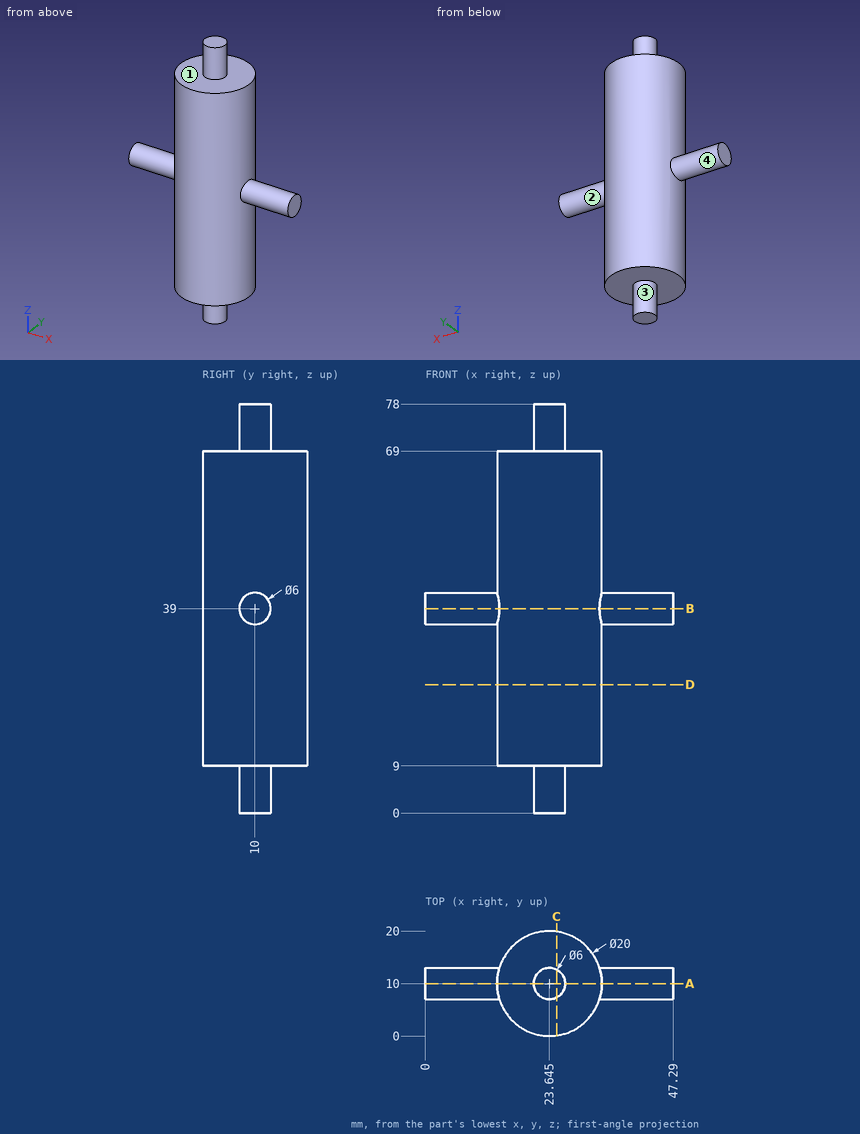
Part print with two shaded views. Sizes in mm from the minimum x, y, z corner. A direction names the side the tool comes from. Coordinates: 2 decimals unless noted, no trailing zeros. Loops run counter-clockwise (first coordinate to the right, second up) from the corner with the lowest first, then second, coordinate; pieces in that order, holes last. Notation, with made-up numbers: (65, -17) - (91, -17) arc R12 cw to (91, -9) - close; hole circle Ø11 at (-16.75, 71). An arc over 180 degrees is marked (long way). Write each question's results on one line, items separated by ' | '. Start each with the question number.
Q1. Slice it at A-A on y = 10. Give the cut face in (x, z) (3 decimals).
Q2. Slice it at D-D on z = 24.5. Give the cut face in (x, y) (3 decimals).
Q3. Drop flat-ended pins along their axis: pin 1 Ø1 at (y, z) = (11, 26.5) entering from +X; pin 2 Ø3 at (x, z) = (13.5, 54.5) entering from +Y; pin 3 Ø5 at (x, y) = (34, 3.5) entering from -Z; pin 4 Ø10 at (x, y) = (30.5, 13.5) entering from +Z. Give the stop position or say it passes through.
Q4. Slice it at B-B on z = 39. Give the cut face in (x, y) (3 decimals), and give its area (3 significant figures).
Q5. Slice it at C-C on x = 25. Give the cut face in (y, z), and give its area (3 significant figures).
Q6. Which spindle directions (+Z, -Z, +X, -X, +Y, -Y) get a long thin tool onto all of the face, cutting with end or side? Do the marked faces 1, 2, 3 and 4. Say none if no direction does.
Q7. Probe line 1 along Z through (x, y) = (16, 11.5); line 2 along Y through (x, z) = (15.5, 61); line 3 along X through (y, z) = (11, 8.5). List the from-to ranges inside material, lowest first.
Answer:
1) outline: (0, 36) - (13.645, 36) - (13.645, 9) - (20.645, 9) - (20.645, 0) - (26.645, 0) - (26.645, 9) - (33.645, 9) - (33.645, 36) - (47.29, 36) - (47.29, 42) - (33.645, 42) - (33.645, 69) - (26.645, 69) - (26.645, 78) - (20.645, 78) - (20.645, 69) - (13.645, 69) - (13.645, 42) - (0, 42) - close
2) outline: circle Ø20 at (23.645, 10)
3) pin 1: stops at x = 33.63 | pin 2: stops at y = 15.03 | pin 3: stops at z = 9 | pin 4: stops at z = 78
4) outline: (0, 7) - (14.106, 7) arc R10 ccw to (33.184, 7) - (47.29, 7) - (47.29, 13) - (33.184, 13) arc R10 ccw to (14.106, 13) - (0, 13) - close | area: 480 mm2
5) outline: (0.09, 9) - (7.32, 9) - (7.32, 0) - (12.68, 0) - (12.68, 9) - (19.91, 9) - (19.91, 69) - (12.68, 69) - (12.68, 78) - (7.32, 78) - (7.32, 69) - (0.09, 69) - close | area: 1,290 mm2
6) face 1: +Z | face 2: +X | face 3: -Z | face 4: -X
7) line 1: z = 9 to 69 | line 2: y = 4.2 to 15.8 | line 3: x = 20.82 to 26.47
